Part model, mm, in its own coordinate system. Face numbers are marked on the shaded views. A direction names the side the tool comes from. Round coordinates to 2 decimals unless told otherwise and drop trailing zeros. Order: outer loops, then holes, each group sorted by start corner. A loop starts at its lowest first (then second) coordinate and runs counter-clockwise, first axis right, second up. Notation, with made-up numbers: (44, -11) -> (77, -11) arc R20 ccw to (77, 26) -> close; hole circle Ø5 at (-9, 84.5). An arc over 180 degrees is marked (long way). Use CSV: the item, a comma, the result in double quotes.
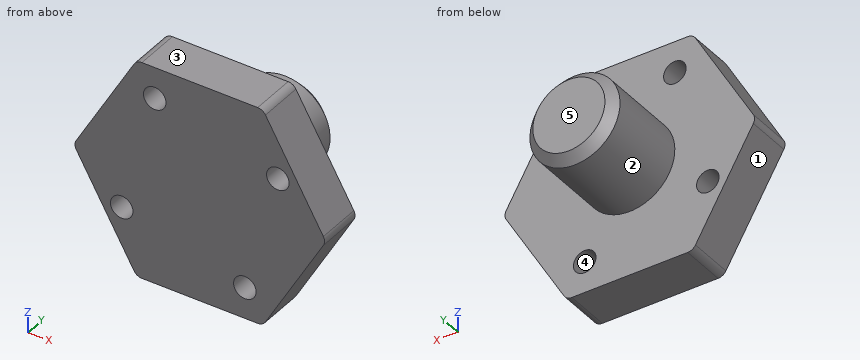
```python
from build123d import *

# Parameters (mm, degrees)
SKETCH_1_R      = 1.25
EXTRUDE_1_DEPTH = 5
SKETCH_2_R      = 5
EXTRUDE_2_DEPTH = 10
FILLET_1_R      = 1
CHAMFER_1_SIZE  = 1


with BuildPart() as part:
    # Эскиз1 → Бобышка-Вытянуть1 (new body)
    with BuildSketch(Plane(origin=(0, 0, 0), x_dir=(1, 0, 0), z_dir=(0, 1, 0))):
        Polygon((14, 0), (7, 12.124355653), (-7, 12.124355653), (-14, 0), (-7, -12.124355653), (7, -12.124355653), align=None)
        with Locations(Location((5, 8.660254038, 0), (0, 0, 270))):
            Circle(SKETCH_1_R, mode=Mode.SUBTRACT)
        with Locations(Location((8.660254038, -5, 0), (0, 0, 270))):
            Circle(SKETCH_1_R, mode=Mode.SUBTRACT)
        with Locations(Location((-5, -8.660254038, 0), (0, 0, 270))):
            Circle(SKETCH_1_R, mode=Mode.SUBTRACT)
        with Locations(Location((-8.660254038, 5, 0), (0, 0, 270))):
            Circle(SKETCH_1_R, mode=Mode.SUBTRACT)
    extrude(amount=EXTRUDE_1_DEPTH)

    # Эскиз2 → Бобышка-Вытянуть2 (add)
    with BuildSketch(Plane(origin=(0, 5, 0), x_dir=(1, 0, 0), z_dir=(0, 1, 0))):
        with Locations(Location((0, 0, 0), (0, 0, 270))):
            Circle(SKETCH_2_R)
    extrude(amount=EXTRUDE_2_DEPTH)

    # Скругление1
    fillet_1_edges = [part.edges().sort_by_distance(p)[0] for p in [
        (7, 2.5, 12.124355653),
        (-7, 2.5, 12.124355653),
        (-14, 2.5, 0),
        (-7, 2.5, -12.124355653),
        (7, 2.5, -12.124355653),
        (14, 2.5, 0),
    ]]
    fillet(fillet_1_edges, radius=FILLET_1_R)

    # Фаска1
    chamfer_1_edges = [part.edges().sort_by_distance(p)[0] for p in [
        (0, 15, -5),
    ]]
    chamfer(chamfer_1_edges, length=CHAMFER_1_SIZE)


solid = part.part
```
(1) Pull direction Z, two halves, no side cores. Call the marked faces 3, 4 and 5: released by +Z, released by -Z, zero draft, split by the parting line, or undercut.
Reply:
face 3,"released by +Z"
face 4,"undercut"
face 5,"zero draft"
(2) Cut at B-B, the plane z = 0. Give the cut face in (x, y), then the cut area to 3 significant figures.
Reply:
outline,"(-13.85, 0) -> (13.85, 0) -> (13.85, 5) -> (5, 5) -> (5, 14) -> (4, 15) -> (-4, 15) -> (-5, 14) -> (-5, 5) -> (-13.85, 5) -> close"
area,"237 mm2"
(3) Cut at A-A, the plane x = -5.5. Give the cut face in (y, z), then the cut area to 3 significant figures.
Reply:
outline,"(0, -12.12) -> (5, -12.12) -> (5, 7.51) -> (0, 7.51) -> close; (0, 9.81) -> (5, 9.81) -> (5, 12.12) -> (0, 12.12) -> close"
area,"110 mm2"
(4) Cut at C-C, the plane y = 2.25. Give the cut face in (x, z).
Reply:
outline,"(-13.71, -0.5) -> (-7.29, -11.62) arc R1 ccw to (-6.42, -12.12) -> (6.42, -12.12) arc R1 ccw to (7.29, -11.62) -> (13.71, -0.5) arc R1 ccw to (13.71, 0.5) -> (7.29, 11.62) arc R1 ccw to (6.42, 12.12) -> (-6.42, 12.12) arc R1 ccw to (-7.29, 11.62) -> (-13.71, 0.5) arc R1 ccw to start; hole circle Ø2.5 at (-8.66, -5); hole circle Ø2.5 at (-5, 8.66); hole circle Ø2.5 at (5, -8.66); hole circle Ø2.5 at (8.66, 5)"
(5) Which spindle directions (+Z, -Z, +X, -X, +Y, -Y) get a long thin tool onto all of the face, cutting with end or side? Do the marked faces 1 and 2. Say none if no direction does.
Reply:
face 1,"-Z, -X, +Y, -Y"
face 2,"+Y"
(6) Cut at D-D, the plane z = 5.75. Give the cut face in (x, y).
Reply:
outline,"(-10.68, 0) -> (7.66, 0) -> (7.66, 5) -> (-10.68, 5) -> close; (9.66, 0) -> (10.68, 0) -> (10.68, 5) -> (9.66, 5) -> close"
(7) Drop flat-ended pins along their axis: P1, Ø3, axis at x = 8.66, z = 5, coming from the +Y side; P2, Ø8, axis at x = -7, y = 12.5, coming from the +Z side; P3, Ø2, axis at x = -8.66, z = -5, coming from the +Y side; P4, Ø2, axis at x = -7.5, z = 9.5, coming from the -Y side. Give the stop position or say it passes through.
Reply:
P1,"y = 5"
P2,"z = 4"
P3,"through"
P4,"y = 0"
(8) Probe probe 1 along Y at (x, z) = (-6.75, -9.5); probe 2 along X at (y, z) = (1.25, -5); probe 3 along X at (y, z) = (3.5, 5). List the from-to ranges inside material, lowest first. Write a range as [from, to].
Reply:
probe 1,"[0, 5]"
probe 2,"[-11.11, -9.91], [-7.41, 11.11]"
probe 3,"[-11.11, 7.41], [9.91, 11.11]"
